```python
from build123d import *

# Parameters (mm, degrees)
F0_W     = 51
F0_H     = 5
F0_W_2   = 1.5
F0_H_2   = 1.5
F1_DEPTH = 8.5


with BuildPart() as f1:
    # F0 (on Top) → F1 (new body)
    with BuildSketch(Plane.XY):
        with Locations((25.5, 2.5)):
            Rectangle(F0_W, F0_H)
        with Locations((1.95, 1.25)):
            Rectangle(F0_W_2, F0_H_2, mode=Mode.SUBTRACT)
        with Locations((4.42, 1.25)):
            Rectangle(F0_W_2, F0_H_2, mode=Mode.SUBTRACT)
        with Locations((6.89, 1.25)):
            Rectangle(F0_W_2, F0_H_2, mode=Mode.SUBTRACT)
        with Locations((9.36, 1.25)):
            Rectangle(F0_W_2, F0_H_2, mode=Mode.SUBTRACT)
        with Locations((11.83, 1.25)):
            Rectangle(F0_W_2, F0_H_2, mode=Mode.SUBTRACT)
        with Locations((14.3, 1.25)):
            Rectangle(F0_W_2, F0_H_2, mode=Mode.SUBTRACT)
        with Locations((16.77, 1.25)):
            Rectangle(F0_W_2, F0_H_2, mode=Mode.SUBTRACT)
        with Locations((19.24, 1.25)):
            Rectangle(F0_W_2, F0_H_2, mode=Mode.SUBTRACT)
        with Locations((21.71, 1.25)):
            Rectangle(F0_W_2, F0_H_2, mode=Mode.SUBTRACT)
        with Locations((24.18, 1.25)):
            Rectangle(F0_W_2, F0_H_2, mode=Mode.SUBTRACT)
        with Locations((26.65, 1.25)):
            Rectangle(F0_W_2, F0_H_2, mode=Mode.SUBTRACT)
        with Locations((29.12, 1.25)):
            Rectangle(F0_W_2, F0_H_2, mode=Mode.SUBTRACT)
        with Locations((31.59, 1.25)):
            Rectangle(F0_W_2, F0_H_2, mode=Mode.SUBTRACT)
        with Locations((34.06, 1.25)):
            Rectangle(F0_W_2, F0_H_2, mode=Mode.SUBTRACT)
        with Locations((36.53, 1.25)):
            Rectangle(F0_W_2, F0_H_2, mode=Mode.SUBTRACT)
        with Locations((39, 1.25)):
            Rectangle(F0_W_2, F0_H_2, mode=Mode.SUBTRACT)
        with Locations((41.47, 1.25)):
            Rectangle(F0_W_2, F0_H_2, mode=Mode.SUBTRACT)
        with Locations((43.94, 1.25)):
            Rectangle(F0_W_2, F0_H_2, mode=Mode.SUBTRACT)
        with Locations((46.41, 1.25)):
            Rectangle(F0_W_2, F0_H_2, mode=Mode.SUBTRACT)
        with Locations((48.88, 1.25)):
            Rectangle(F0_W_2, F0_H_2, mode=Mode.SUBTRACT)
        with Locations((1.95, 3.75)):
            Rectangle(F0_W_2, F0_H_2, mode=Mode.SUBTRACT)
        with Locations((4.42, 3.75)):
            Rectangle(F0_W_2, F0_H_2, mode=Mode.SUBTRACT)
        with Locations((6.89, 3.75)):
            Rectangle(F0_W_2, F0_H_2, mode=Mode.SUBTRACT)
        with Locations((9.36, 3.75)):
            Rectangle(F0_W_2, F0_H_2, mode=Mode.SUBTRACT)
        with Locations((11.83, 3.75)):
            Rectangle(F0_W_2, F0_H_2, mode=Mode.SUBTRACT)
        with Locations((14.3, 3.75)):
            Rectangle(F0_W_2, F0_H_2, mode=Mode.SUBTRACT)
        with Locations((16.77, 3.75)):
            Rectangle(F0_W_2, F0_H_2, mode=Mode.SUBTRACT)
        with Locations((19.24, 3.75)):
            Rectangle(F0_W_2, F0_H_2, mode=Mode.SUBTRACT)
        with Locations((21.71, 3.75)):
            Rectangle(F0_W_2, F0_H_2, mode=Mode.SUBTRACT)
        with Locations((24.18, 3.75)):
            Rectangle(F0_W_2, F0_H_2, mode=Mode.SUBTRACT)
        with Locations((26.65, 3.75)):
            Rectangle(F0_W_2, F0_H_2, mode=Mode.SUBTRACT)
        with Locations((29.12, 3.75)):
            Rectangle(F0_W_2, F0_H_2, mode=Mode.SUBTRACT)
        with Locations((31.59, 3.75)):
            Rectangle(F0_W_2, F0_H_2, mode=Mode.SUBTRACT)
        with Locations((34.06, 3.75)):
            Rectangle(F0_W_2, F0_H_2, mode=Mode.SUBTRACT)
        with Locations((36.53, 3.75)):
            Rectangle(F0_W_2, F0_H_2, mode=Mode.SUBTRACT)
        with Locations((39, 3.75)):
            Rectangle(F0_W_2, F0_H_2, mode=Mode.SUBTRACT)
        with Locations((41.47, 3.75)):
            Rectangle(F0_W_2, F0_H_2, mode=Mode.SUBTRACT)
        with Locations((43.94, 3.75)):
            Rectangle(F0_W_2, F0_H_2, mode=Mode.SUBTRACT)
        with Locations((46.41, 3.75)):
            Rectangle(F0_W_2, F0_H_2, mode=Mode.SUBTRACT)
        with Locations((48.88, 3.75)):
            Rectangle(F0_W_2, F0_H_2, mode=Mode.SUBTRACT)
    extrude(amount=F1_DEPTH)


solid = f1.part
```
The model under review builds one solid part; all positions refer to its coordinate system, in mm. Coordinates: 2 decimals unless noted, no trailing zeros. Write each loop counter-clockwise with the first axis right and the second up, starting at its lowest first coordinate (ties: lowest second). Pieces come first, ordered by that corner, then holes. Notation, with made-up numbers: (-2, 84.25) -> (31, 84.25) arc R16 ccw to (31, 96.25) -> close; hole circle Ø10 at (77, 77). An arc over 180 degrees is marked (long way). One line per item, written item: value. Start each with the question number.
Q1. Add section A-A, the plane x = 44. Give the boundary of the cut face in (y, z).
Q2. Add section B-B, the plane y = 3.5. Count the separate pieces of the cut face and the enclosed holes in it, then the cut area to 4 significant figures.
Q3. Clearance check with a flat-ended pin moving along its axis: P1, Ø1.2, axis at y = 1.5, z = 5, coming from the -X side. State where the tip first meets the part, or that it passes through.
Q4. The part is to be moulded in two halves that separate along X. For faces 1 (the face through (17.52, 4, 4)), 2 (the face through (25.1, 2.5, 0)), say which applies: +X half, -X half, draft (parallel to the pull), parting line (faces both ways), or undercut.
Q5. To check wall thickness, follow probe 1 along Y at (x, z) = (26, 4). State the ranges of the line that lie inside material, in increasing order.
Response:
1. outline: (0, 0) -> (0.5, 0) -> (0.5, 8.5) -> (0, 8.5) -> close; (2, 0) -> (3, 0) -> (3, 8.5) -> (2, 8.5) -> close; (4.5, 0) -> (5, 0) -> (5, 8.5) -> (4.5, 8.5) -> close
2. separate pieces: 21
2. enclosed holes: 0
2. area: 178.5 mm²
3. P1: x = 0
4. face 1: undercut
4. face 2: draft
5. probe 1: 0 to 0.5, 2 to 3, 4.5 to 5
